The figure shows three views and two pictorial views of one solid part (mm, origin at its lowest corner). Answer the questions. A direction names the side the tool comes from. Give positions to 0.01 mm unless a question says otherwise; leave off trailing zeros. Write each loop counter-clockwise with the first axis right and the second up, starting at its lowest first coordinate (ties: lowest second). Pieces come first, ordered by that corner, then holes. Notation, with made-up numbers: M 38,45.5 L 80,45.5 A14 ccw 80,52.5 Z; hole C 13,-39.5 d6. An arc over 180 degrees is marked long. Return JSON: item names as keys, results as strings.
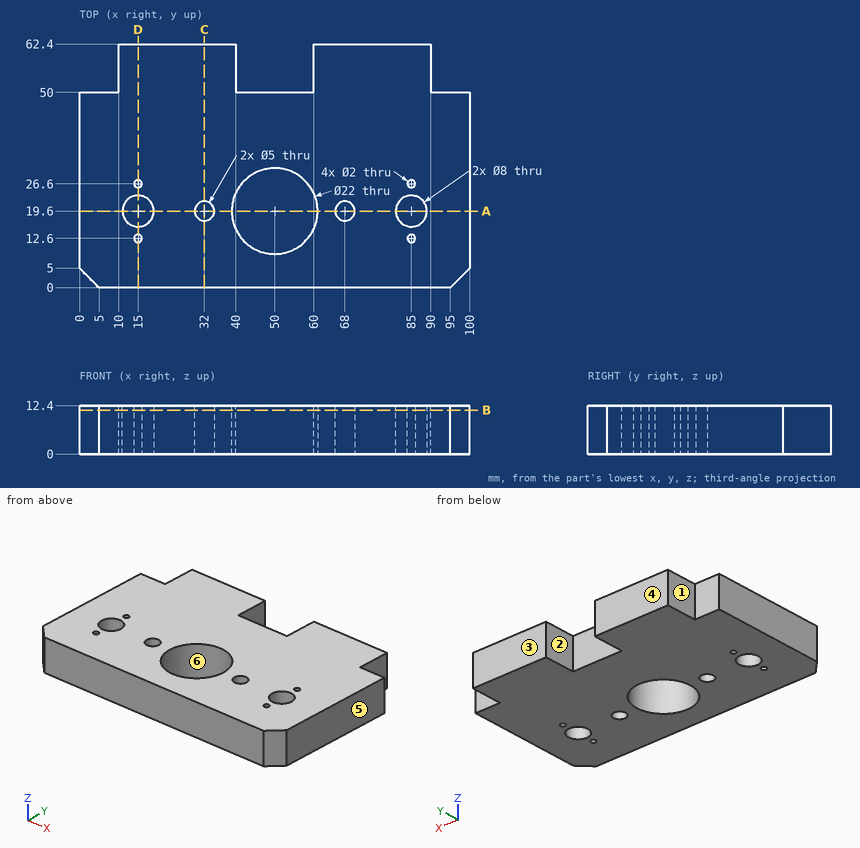
Item 1: Which of the six approach directions +Z, -Z, +X, -X, +Y, -Y give full straight-line access (tool end or side, diameter ignored) to the marked faces 1, 2 and 3?
Geometry results:
{"face 1": "+Z, -Z, -X, +Y", "face 2": "+Z, -Z, +Y", "face 3": "+Z, -Z, +X, -X, +Y"}
Item 2: A cutting plane is placed at C-C, the plane x = 32. Write down the section's boundary in (y, z).
Geometry results:
{"outline": "M 0,0 L 17.1,0 L 17.1,12.4 L 0,12.4 Z; M 22.1,0 L 62.4,0 L 62.4,12.4 L 22.1,12.4 Z"}
Item 3: Determine the mould class of the marked faces 4, 5 and 6 for opening direction X: +X half, -X half, draft (parallel to the pull), parting line (faces both ways), or undercut.
Geometry results:
{"face 4": "draft", "face 5": "+X half", "face 6": "undercut"}
Item 4: Given pin 1 Ø13 at (x, y) = (50, 19.6) entering from -Z; pin 2 Ø3.5 at (y, z) = (56, 3) entering from -X; pin 3 Ø3.5 at (y, z) = (55, 8) entering from +X; pin 4 Ø6 at (x, z) = (46, 3.5) entering from +Y, each flat-ended and moving along its own axis, determine where each tip first touches the part or whether it passes through.
Geometry results:
{"pin 1": "passes through", "pin 2": "stops at x = 10", "pin 3": "stops at x = 90", "pin 4": "stops at y = 50"}
Item 5: Find the intervals of material crossed by line 1 (Y direction, x = 15, z = 6.25); line 2 (X direction, y = 19.6, z = 7); line 3 (Y direction, x = 32, z = 8.5), in increasing order.
Geometry results:
{"line 1": "y = 0 to 11.6, 13.6 to 15.6, 23.6 to 25.6, 27.6 to 62.4", "line 2": "x = 0 to 11, 19 to 29.5, 34.5 to 39, 61 to 65.5, 70.5 to 81, 89 to 100", "line 3": "y = 0 to 17.1, 22.1 to 62.4"}
Item 6: A cutting plane is placed at D-D, the plane x = 15. Write down the section's boundary in (y, z).
Geometry results:
{"outline": "M 0,0 L 11.6,0 L 11.6,12.4 L 0,12.4 Z; M 13.6,0 L 15.6,0 L 15.6,12.4 L 13.6,12.4 Z; M 23.6,0 L 25.6,0 L 25.6,12.4 L 23.6,12.4 Z; M 27.6,0 L 62.4,0 L 62.4,12.4 L 27.6,12.4 Z"}
Item 7: A cutting plane is placed at A-A, the plane y = 19.6. Write down the section's boundary in (x, z), plus the area to 3 significant figures.
Geometry results:
{"outline": "M 0,0 L 11,0 L 11,12.4 L 0,12.4 Z; M 19,0 L 29.5,0 L 29.5,12.4 L 19,12.4 Z; M 34.5,0 L 39,0 L 39,12.4 L 34.5,12.4 Z; M 61,0 L 65.5,0 L 65.5,12.4 L 61,12.4 Z; M 70.5,0 L 81,0 L 81,12.4 L 70.5,12.4 Z; M 89,0 L 100,0 L 100,12.4 L 89,12.4 Z", "area": "645 mm2"}
Item 8: A cutting plane is placed at B-B, the plane z = 11.25. Count the separate pieces of the cut face and the enclosed holes in it, plus the area to 3 significant figures.
Geometry results:
{"separate pieces": "1", "enclosed holes": "9", "area": "5,190 mm2"}
